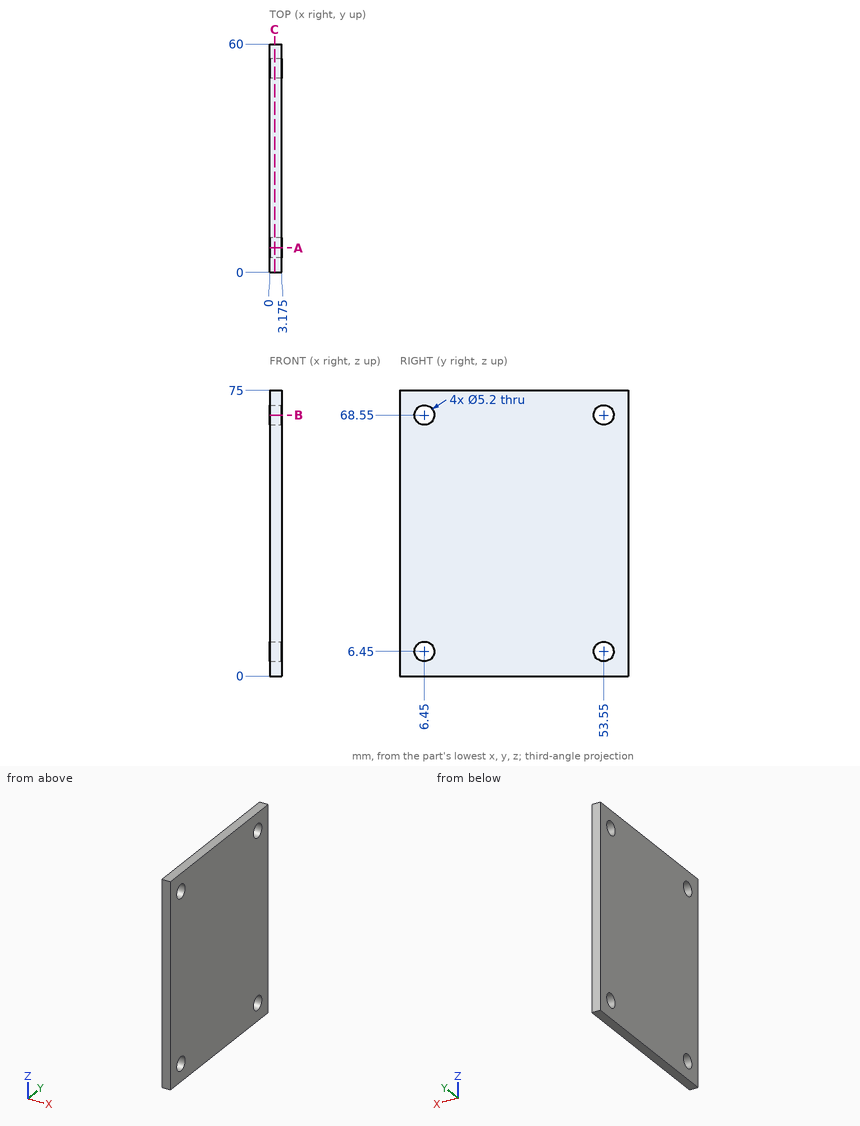
Check sheet for the drawn part. Datum: minimum x, y, z corner. Units: mm. Coordinates: 2 decimals unless noted, no trailing zeros. Loops run counter-clockwise (first coordinate to the right, second up) from the corner with the lowest first, then second, coordinate; pieces in that order, holes last. Notation, with made-up numbers: (-11, -4) -> (26, -4) arc R14 cw to (26, 13) -> close; hole circle Ø4 at (-12, 36.5). An arc over 180 degrees is marked (long way). Answer as a JSON object with one key per item and string values. Group by question number.
Item 1: Sectioned sample at A-A on y = 6.45. Record the boundary of the cut face in (x, z) (3 decimals), plus the area to 3 significant figures.
Item 2: Scan lines: probe 1 along Y at (x, z) = (1.5, 6.45); probe 2 along Y at (x, z) = (1.35, 5). Record each from-to range of solid material in increasing order.
Item 3: Sectioned sample at B-B on z = 68.55. Record the boundary of the cut face in (x, y) (3 decimals), plus the area to 3 significant figures.
Item 4: Sectioned sample at C-C on x = 1.3. Record the boundary of the cut face in (y, z).
Evaluation:
{
 "1": {"outline": "(0, 0) -> (3.175, 0) -> (3.175, 3.85) -> (0, 3.85) -> close; (0, 9.05) -> (3.175, 9.05) -> (3.175, 65.95) -> (0, 65.95) -> close; (0, 71.15) -> (3.175, 71.15) -> (3.175, 75) -> (0, 75) -> close", "area": "205 mm²"},
 "2": {"probe 1": "y = 0 to 3.85, 9.05 to 50.95, 56.15 to 60", "probe 2": "y = 0 to 4.29, 8.61 to 51.39, 55.71 to 60"},
 "3": {"outline": "(0, 0) -> (3.175, 0) -> (3.175, 3.85) -> (0, 3.85) -> close; (0, 9.05) -> (3.175, 9.05) -> (3.175, 50.95) -> (0, 50.95) -> close; (0, 56.15) -> (3.175, 56.15) -> (3.175, 60) -> (0, 60) -> close", "area": "157 mm²"},
 "4": {"outline": "(0, 0) -> (60, 0) -> (60, 75) -> (0, 75) -> close; hole circle Ø5.2 at (6.45, 6.45); hole circle Ø5.2 at (6.45, 68.55); hole circle Ø5.2 at (53.55, 6.45); hole circle Ø5.2 at (53.55, 68.55)"}
}
